```python
from build123d import *

# Parameters (mm, degrees)
F1_DEPTH = 15
F2_T     = -1.2
F3_R     = 5
F4_R     = 5


with BuildPart() as f1:
    # F0 (on Top) → F1 (new body)
    with BuildSketch(Plane.XY):
        with BuildLine():
            Line((35.3129135817, 42.7640778485), (-107.1870864183, 42.7640778485))
            ThreePointArc((-107.1870864183, 42.7640778485), (-114.2581542301, 39.8351456603), (-117.1870864183, 32.7640778485))
            Line((-117.1870864183, 32.7640778485), (-117.1870864183, -39.7359221515))
            ThreePointArc((-117.1870864183, -39.7359221515), (-114.2581542301, -46.8069899634), (-107.1870864183, -49.7359221515))
            Line((-107.1870864183, -49.7359221515), (35.3129135817, -49.7359221515))
            ThreePointArc((35.3129135817, -49.7359221515), (42.3839813936, -46.8069899634), (45.3129135817, -39.7359221515))
            Line((45.3129135817, -39.7359221515), (45.3129135817, 32.7640778485))
            ThreePointArc((45.3129135817, 32.7640778485), (42.3839813936, 39.8351456603), (35.3129135817, 42.7640778485))
        make_face()
    extrude(amount=F1_DEPTH)

    # F2
    f2_openings = [f1.faces().sort_by_distance(p)[0] for p in [
        (-35.937086, -3.485922, 15),
    ]]
    offset(amount=F2_T, openings=f2_openings)

    # F3
    f3_edges = [f1.edges().sort_by_distance(p)[0] for p in [
        (-35.937086, 41.564078, 1.2),
        (-113.409626, 38.986618, 1.2),
        (-115.987086, -3.485922, 1.2),
        (-113.409626, -45.958462, 1.2),
        (-35.937086, -48.535922, 1.2),
        (41.535453, -45.958462, 1.2),
        (44.112914, -3.485922, 1.2),
        (41.535453, 38.986618, 1.2),
    ]]
    fillet(f3_edges, radius=F3_R)

    # F4
    f4_edges = [f1.edges().sort_by_distance(p)[0] for p in [
        (-35.937086, 42.764078, 0),
        (-114.258154, 39.835146, 0),
        (-117.187086, -3.485922, 0),
        (-114.258154, -46.80699, 0),
        (-35.937086, -49.735922, 0),
        (42.383981, -46.80699, 0),
        (45.312914, -3.485922, 0),
        (42.383981, 39.835146, 0),
    ]]
    fillet(f4_edges, radius=F4_R)


solid = f1.part
```
Input: part model. Units: mm. Frame: model coordinates. A direction names the side the tool comes from. Give positions to 0.01 mm unless a question says otherwise; leave off trailing zeros. Order: outer loops, then holes, each group sorted by start corner. A loop starts at its lowest first (then second) coordinate and runs counter-clockwise, first axis right, second up. Notation, with made-up numbers: M -28.75,29 L -1.75,29 A16 ccw -1.75,35 Z; hole C -5.5,21 d5. An arc over 180 degrees is marked long. Return JSON: item names as keys, results as strings.
Item 1: Cut plane A-A (z = 8). Return loops of the section in (x, y), then the cut area to 3 significant figures.
Solutions:
{"outline": "M -117.19,-39.74 A10 ccw -107.19,-49.74 L 35.31,-49.74 A10 ccw 45.31,-39.74 L 45.31,32.76 A10 ccw 35.31,42.76 L -107.19,42.76 A10 ccw -117.19,32.76 Z; hole M -115.99,-39.74 A8.8 ccw -107.19,-48.54 L 35.31,-48.54 A8.8 ccw 44.11,-39.74 L 44.11,32.76 A8.8 ccw 35.31,41.56 L -107.19,41.56 A8.8 ccw -115.99,32.76 Z", "area": "587 mm^2"}
Item 2: Cut plane C-C (x = -53). Return loops of the section in (y, z).
Solutions:
{"outline": "M -49.74,5 A5 ccw -44.74,0 L 37.76,0 A5 ccw 42.76,5 L 42.76,15 L 41.56,15 L 41.56,6.2 A5 cw 36.56,1.2 L -43.54,1.2 A5 cw -48.54,6.2 L -48.54,15 L -49.74,15 Z"}
Item 3: Pull-direction query (Y, two-part tool) for faces 1 (the flat face through (-37, -48.536, 11)), 2 (the flat face through (-35, 42.764, 10)), 3 (the flat face through (45.313, -4, 10)), 4 (the cylindrical face through (42.31, -46.88, 9.93)); classes: +Y half, -Y half, draft (parallel to the pull), parting line (faces both ways), or undercut.
Solutions:
{"face 1": "undercut", "face 2": "+Y half", "face 3": "draft", "face 4": "-Y half"}
Item 4: Cut plane B-B (y = -38). Return loops of the section in (x, z).
Solutions:
{"outline": "M -117.19,5 A5 ccw -112.19,0 L 40.31,0 A5 ccw 45.31,5 L 45.31,15 L 44.11,15 L 44.11,6.2 A5 cw 39.11,1.2 L -110.99,1.2 A5 cw -115.99,6.2 L -115.99,15 L -117.19,15 Z"}
Item 5: Access query for faces 5 (the cylindrical face through (-115.76, -3.99, 1.5)), 6 (the flat face through (44.113, -4, 11)). Directions: +Z, -Z, +X, -X, +Y, -Y. A direction counts if a zero-diameter tool reaches every point of the face in a straight line with its end or side. Return the directions, or none.
Solutions:
{"face 5": "-Z, -X, +Y, -Y", "face 6": "+Z"}
Item 6: Ray query, probe 1 along X at (y, z) = (-34, 9); probe 2 along Y at (x, z) = (32.5, 9); probe 3 along Z at (x, y) = (-92.5, 32). Return the intervals inside material, ascending.
Solutions:
{"probe 1": "-117.19 to -115.99, 44.11 to 45.31", "probe 2": "-49.74 to -48.54, 41.56 to 42.76", "probe 3": "0 to 1.2"}
